For this review, take the finished solid that the model builds, in its own axes (mm). A direction names the side the tool comes from. Give positions to 0.01 mm unless a question says otherwise; leave off trailing zeros. Loops run counter-clockwise (first coordinate to the right, second up) from the corner with the lowest first, then second, coordinate; pieces in that order, holes last. Notation, with made-up numbers: (59, 8) - (96, 8) arc R14 cw to (96, 23) - close; hole circle Ø5 at (40.5, -31). An arc over 180 degrees is marked (long way). Put each result on its own line as item: value.
from build123d import *

# Parameters (mm, degrees)
SKETCH1_W                                           = 101.6
SKETCH1_H                                           = 82.55
BOSS_EXTRUDE1_DEPTH                                 = 15.875
SKETCH2_W                                           = 101.6
SKETCH2_H                                           = 2.55
CUT_EXTRUDE1_DEPTH                                  = 100.943496537
CBORE_FOR_M8_HEX_SOCKET_HEAD_CAP_SCREW1_D           = 9
CBORE_FOR_M8_HEX_SOCKET_HEAD_CAP_SCREW1_CBORE_D     = 15
CBORE_FOR_M8_HEX_SOCKET_HEAD_CAP_SCREW1_CBORE_DEPTH = 9


with BuildPart() as part:
    # Sketch1 → Boss-Extrude1 (new, symmetric)
    with BuildSketch(Plane.XY):
        with Locations((0, 38.725)):
            Rectangle(SKETCH1_W, SKETCH1_H)
    extrude(amount=BOSS_EXTRUDE1_DEPTH, both=True)

    # Sketch2 → Cut-Extrude1 (cut, through all)
    with BuildSketch(Plane.XY.offset(15.875)):
        with Locations((0, -1.275)):
            Rectangle(SKETCH2_W, SKETCH2_H)
    extrude(amount=-CUT_EXTRUDE1_DEPTH, mode=Mode.SUBTRACT)

    # CBORE for M8 Hex Socket Head Cap Screw1 (through all)
    with Locations(Plane(origin=(0, 80, 0), x_dir=(1, 0, 0), z_dir=(0, 1, 0))):
        with Locations((30, 0), (0, 0), (-30, 0)):
            CounterBoreHole(CBORE_FOR_M8_HEX_SOCKET_HEAD_CAP_SCREW1_D / 2, CBORE_FOR_M8_HEX_SOCKET_HEAD_CAP_SCREW1_CBORE_D / 2, CBORE_FOR_M8_HEX_SOCKET_HEAD_CAP_SCREW1_CBORE_DEPTH)


solid = part.part
1) Wall thickness on line 1 (Z direction, x = 30, y = 23.5) (3 decimals); line 2 (Z direction, x = 30, y = 75.25) (3 decimals); line 3 (X direction, y = 8, z = -2.5): over which ranges is each line inside the solid? List them lowest first.
Geometry check:
line 1: z = -15.875 to -4.5, 4.5 to 15.875
line 2: z = -15.875 to -7.5, 7.5 to 15.875
line 3: x = -50.8 to -33.74, -26.26 to -3.74, 3.74 to 26.26, 33.74 to 50.8
2) For faces 1 (the face through (25.708, 35.003, -1.352)), 2 (the face through (22.507, 75.563, -0.33)), list the 3-axis set-ups (+Z, -Z, +X, -X, +Y, -Y) from which the entire face can be reached by the end or side of a thin tool; tool diameter is ignored.
Geometry check:
face 1: +Y, -Y
face 2: +Y
3) Take a section at A-A on z = 0. State the section outline as (x, y) points, and give its area (3 significant figures).
Geometry check:
outline: (-50.8, 0) - (-34.5, 0) - (-34.5, 71) - (-37.5, 71) - (-37.5, 80) - (-50.8, 80) - close; (-25.5, 0) - (-4.5, 0) - (-4.5, 71) - (-7.5, 71) - (-7.5, 80) - (-22.5, 80) - (-22.5, 71) - (-25.5, 71) - close; (4.5, 0) - (25.5, 0) - (25.5, 71) - (22.5, 71) - (22.5, 80) - (7.5, 80) - (7.5, 71) - (4.5, 71) - close; (34.5, 0) - (50.8, 0) - (50.8, 80) - (37.5, 80) - (37.5, 71) - (34.5, 71) - close
area: 5,810 mm²
4) Draft analysis for pull direction Z (two halves, no side actions). For faces 3 (the face through (-1, 41, 15.875)), 4 (the face through (0, 71, 5)), 5 (the face through (-50.8, 39, 0)), 6 (the face through (-1, 41, -15.875)), state which applies: pulls with the +Z half, pulls with the -Z half, needs draft (parallel to the pull), parting line crosses it, or undercut.
Geometry check:
face 3: pulls with the +Z half
face 4: undercut
face 5: needs draft
face 6: pulls with the -Z half
5) Take a section at D-D on x = 1.5. State the section outline as (y, z) points (3 decimals).
Geometry check:
outline: (0, -15.875) - (80, -15.875) - (80, -7.348) - (71, -7.348) - (71, -4.243) - (0, -4.243) - close; (0, 4.243) - (71, 4.243) - (71, 7.348) - (80, 7.348) - (80, 15.875) - (0, 15.875) - close
6) Insertion check: pin 1 Ø10.5 at (x, z) = (30, 0) entering from +Y; pin 2 Ø8 at (x, z) = (-30, 0) entering from -Y; pin 3 Ø7.5 at (x, z) = (-2.5, -3) entering from +Y. Each pin has a flat end and moves straight along its axis. Give the tip position at first contact, or say it passes through.
Geometry check:
pin 1: stops at y = 71
pin 2: passes through
pin 3: stops at y = 80
7) Take a section at C-C on y = 39. State the section outline as (x, z) points (3 decimals).
Geometry check:
outline: (-50.8, -15.875) - (50.8, -15.875) - (50.8, 15.875) - (-50.8, 15.875) - close; hole circle Ø9 at (-30, 0); hole circle Ø9 at (0, 0); hole circle Ø9 at (30, 0)
8) Take a section at B-B on x = 30. State the section outline as (y, z) points (3 decimals).
Geometry check:
outline: (0, -15.875) - (80, -15.875) - (80, -7.5) - (71, -7.5) - (71, -4.5) - (0, -4.5) - close; (0, 4.5) - (71, 4.5) - (71, 7.5) - (80, 7.5) - (80, 15.875) - (0, 15.875) - close
